CAD build for the part. Positions are in the model's coordinates, mm. A direction names the side the tool comes from. Round coordinates to 2 decimals unless told otherwise and drop trailing zeros. Write each loop counter-clockwise with the first axis right and the second up, starting at its lowest first coordinate (ties: lowest second). Pieces come first, ordered by that corner, then holes. Notation, with made-up numbers: (7, -10.5) -> (16, -10.5) arc R14 ccw to (16, 2.5) -> close; hole circle Ø9 at (56.25, 1). An arc over 180 degrees is marked (long way). Answer in a Markdown table with one row per item. Add a question column.
```python
from build123d import *

# Parameters (mm, degrees)
F0_W     = 818
F0_H     = 70
F1_DEPTH = 35
F2_W     = 70
F2_H     = 35
F3_DEPTH = 35


with BuildPart() as f1:
    # F0 (on Front) → F1 (new body)
    with BuildSketch(Plane.XZ):
        with Locations((2.655625, -181.434033)):
            Rectangle(F0_W, F0_H)
    extrude(amount=-F1_DEPTH)

    # F2 (on face) → F3 (cut)
    with BuildSketch(Plane.XY.offset(-146.434033)):
        with Locations((-199.250098, 17.5)):
            Rectangle(F2_W, F2_H)
    extrude(amount=-F3_DEPTH, mode=Mode.SUBTRACT)


solid = f1.part
```
Item 1: Saw through at A-A on z = -168.5. Give the cut face in (x, y).
Item 2: Two-plate mould, pull along X, no slides. Class faces 1 (the flat face through (-406.344, 17, -182)), 2 (the flat face through (-3, 17, -216.434)), 3 (the flat face through (-200, 18, -181.434)): +X half, -X half, draft (parallel to the pull), parting line (faces both ways), or undercut.
Item 3: Drill centre line: probe 1 along X at (y, z) = (24, -154.5). Where is it in solid material? Low to high.
Item 4: Saw through at C-C on x = -200. Give the cut face in (y, z), then the cut area to 4 significant figures.
Item 5: Saw through at B-B on y = 20.5. Give the cut face in (x, z), then the cut area to 3 significant figures.
Item 6: Tool access for faces 4 (the flat face through (-3, 0, -181)), 5 (the flat face through (-164.25, 17, -164)): list every direction of +Z, -Z, +X, -X, +Y, -Y with a clear straight run to the whole face (end or side of a thin tool).
Item 7: Pin check, flat tip, straight feed: pin 1 (10.5 mm diameter, centred on x = -215, y = 24, fed in from +Z). Stop position of the tip, or through.
Recorded:
| question | item | result |
|---|---|---|
| 1 | outline | (-406.34, 0) -> (-234.25, 0) -> (-234.25, 35) -> (-406.34, 35) -> close; (-164.25, 0) -> (411.66, 0) -> (411.66, 35) -> (-164.25, 35) -> close |
| 2 | face 1 | -X half |
| 2 | face 2 | draft |
| 2 | face 3 | undercut |
| 3 | probe 1 | -406.34 to -234.25, -164.25 to 411.66 |
| 4 | outline | (0, -216.43) -> (35, -216.43) -> (35, -181.43) -> (0, -181.43) -> close |
| 4 | area | 1,225 mm2 |
| 5 | outline | (-406.34, -216.43) -> (411.66, -216.43) -> (411.66, -146.43) -> (-164.25, -146.43) -> (-164.25, -181.43) -> (-234.25, -181.43) -> (-234.25, -146.43) -> (-406.34, -146.43) -> close |
| 5 | area | 54,800 mm2 |
| 6 | face 4 | +Z, -Z, +X, -X, -Y |
| 6 | face 5 | +Z, +Y, -Y |
| 7 | pin 1 | z = -181.43 |
